The figure shows three views and two pictorial views of one solid part (mm, origin at its lowest corner). Answer the questions. Give positions to 0.01 mm unless a question says otherwise; leave off trailing zeros. Write each loop counter-clockwise with the first axis right and the second up, starting at its lowest first coordinate (ties: lowest second). Pieces come first, ordered by that corner, then holes. Notation, with made-up numbers: (44, 70) - (86, 70) arc R17 cw to (86, 89) - close; hole circle Ø5 at (-4.5, -15). An arc over 180 degrees is marked (long way). Use a Markdown table: item, result. Add a question column.
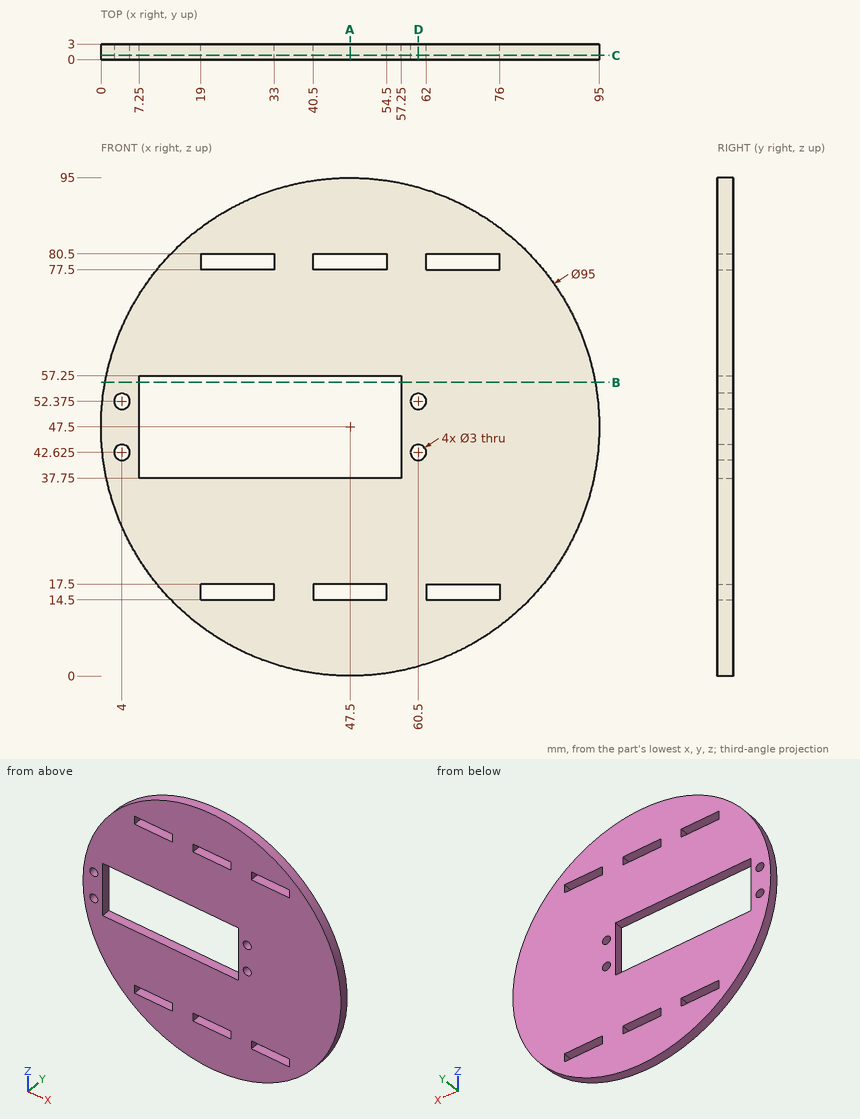
1. Given P1, Ø1, axis at y = 2.5, z = 24.5, coming from the +X side; P2, Ø1.5, axis at x = 48.5, y = 1.5, coming from the -Z side; P3, Ø0.9, axis at y = 2, z = 16.5, coming from the -X side, each flat-ended and moving along its own axis, determine where each tip first touches the part or whether it passes through.
2. Consider L1, parallel to X at y = 0.6, z = 15.5; L2, parallel to X at y = 1.6, z = 47; L3, parallel to Z at x = 60.5, y = 2.15 (3 decimals). Determine where each line is inside the solid, lowest interval first. Write a range as [from, to].
3. The part is cut by section A-A (x = 47.5). Give the vertices of the cut face in (y, z).
4. The part is cut by section B-B (z = 56). Give the vertices of the cut face in (x, y), and give its area (3 significant figures).
5. The part is cut by section D-D (x = 60.5). Give the vertices of the cut face in (y, z) (3 decimals).
6. The part is cut by section C-C (y = 0.85). Count the separate pieces of the cut face and the enclosed holes in it, and give its area (3 significant figures).
Check values:
| question | item | result |
|---|---|---|
| 1 | P1 | stops at x = 89.33 |
| 1 | P2 | stops at z = 0 |
| 1 | P3 | stops at x = 11.13 |
| 2 | L1 | x = [12.4, 19], [33, 40.5], [54.5, 62], [76, 82.6] |
| 2 | L2 | x = [0, 7.25], [57.25, 95] |
| 2 | L3 | z = [1.814, 41.125], [44.125, 50.875], [53.875, 93.186] |
| 3 | outline | (0, 0) - (3, 0) - (3, 14.5) - (0, 14.5) - close; (0, 17.5) - (3, 17.5) - (3, 37.75) - (0, 37.75) - close; (0, 57.25) - (3, 57.25) - (3, 77.5) - (0, 77.5) - close; (0, 80.5) - (3, 80.5) - (3, 95) - (0, 95) - close |
| 4 | outline | (0.77, 0) - (7.25, 0) - (7.25, 3) - (0.77, 3) - close; (57.25, 0) - (94.23, 0) - (94.23, 3) - (57.25, 3) - close |
| 4 | area | 130 mm2 |
| 5 | outline | (0, 1.814) - (3, 1.814) - (3, 41.125) - (0, 41.125) - close; (0, 44.125) - (3, 44.125) - (3, 50.875) - (0, 50.875) - close; (0, 53.875) - (3, 53.875) - (3, 93.186) - (0, 93.186) - close |
| 6 | separate pieces | 1 |
| 6 | enclosed holes | 11 |
| 6 | area | 5,830 mm2 |
